The listing builds one solid part. Answer for the finished solid, in the listing's coordinates (mm). Coordinates: 2 decimals unless noted, no trailing zeros. Loops run counter-clockwise (first coordinate to the right, second up) from the corner with the lowest first, then second, coordinate; pieces in that order, holes last. Notation, with made-up numbers: (60, -32) - (97, -32) arc R7 ccw to (97, -28) - close; hole circle Ø10 at (82.5, -13). An arc over 180 degrees is marked (long way). Put each result on its own line as item: value.
```python
from build123d import *

# Parameters (mm, degrees)
SKETCH1_W           = 31.75
SKETCH1_H           = 38.1
BOSS_EXTRUDE1_DEPTH = 3.175
SKETCH2_R           = 2.15265
CUT_EXTRUDE1_DEPTH  = 42.760604941
SKETCH3_R           = 9.525
CUT_EXTRUDE2_DEPTH  = 42.760604941


with BuildPart() as part:
    # Sketch1 → Boss-Extrude1 (new, symmetric)
    with BuildSketch(Plane(origin=(0, 0, 0), x_dir=(0, 0, -1), z_dir=(1, 0, 0))):
        with Locations((0, 19.05)):
            Rectangle(SKETCH1_W, SKETCH1_H)
    extrude(amount=BOSS_EXTRUDE1_DEPTH, both=True)

    # Sketch2 → Cut-Extrude1 (cut, through all)
    with BuildSketch(Plane(origin=(3.175, 0, 0), x_dir=(0, 0, -1), z_dir=(1, 0, 0))):
        with Locations((-12.7, 3.175)):
            Circle(SKETCH2_R)
        with Locations((-12.7, 34.925)):
            Circle(SKETCH2_R)
        with Locations((12.7, 3.175)):
            Circle(SKETCH2_R)
        with Locations((12.7, 34.925)):
            Circle(SKETCH2_R)
    extrude(amount=-CUT_EXTRUDE1_DEPTH, mode=Mode.SUBTRACT)

    # Sketch3 → Cut-Extrude2 (cut, through all)
    with BuildSketch(Plane(origin=(3.175, 0, 0), x_dir=(0, 0, -1), z_dir=(1, 0, 0))):
        with Locations((0, 19.05)):
            Circle(SKETCH3_R)
    extrude(amount=-CUT_EXTRUDE2_DEPTH, mode=Mode.SUBTRACT)


solid = part.part
```
1) Straight lines are drawn through the part: L1, parallel to Y at x = -1.5, z = -12.7; L2, parallel to Z at x = -2, y = 36.5 (3 decimals); L3, parallel to Z at x = -1.25, y = 36 (3 decimals). For each, find the intervals that lie inside material, in ascending order. Write a range as [from, to].
Found:
L1: y = [0, 1.02], [5.33, 32.77], [37.08, 38.1]
L2: z = [-15.875, -14.167], [-11.233, 11.233], [14.167, 15.875]
L3: z = [-15.875, -14.565], [-10.835, 10.835], [14.565, 15.875]
2) For a pull along Y with two mould halves and no side action, classify faces 1 (the face through (0.04, 9.75, 2.06)), 2 (the face through (0, 38.1, 0)), 3 (the face through (0, 0, 0)), 4 (the face through (0, 19, -15.875)) as pulls with the +Y half, pulls with the -Y half, needs draft (parallel to the pull), parting line crosses it, or undercut.
Found:
face 1: undercut
face 2: pulls with the +Y half
face 3: pulls with the -Y half
face 4: needs draft
3) The part is cut by section B-B (y = 19.05). Give the vertices of the cut face in (x, z) (3 decimals), and give its area (3 significant figures).
Found:
outline: (-3.175, -15.875) - (3.175, -15.875) - (3.175, -9.525) - (-3.175, -9.525) - close; (-3.175, 9.525) - (3.175, 9.525) - (3.175, 15.875) - (-3.175, 15.875) - close
area: 80.6 mm^2
4) The part is cut by section D-D (x = 0.5). Give the vertices of the cut face in (y, z) (3 decimals), and give its area (3 significant figures).
Found:
outline: (0, -15.875) - (38.1, -15.875) - (38.1, 15.875) - (0, 15.875) - close; hole circle Ø4.305 at (3.175, -12.7); hole circle Ø4.305 at (3.175, 12.7); hole circle Ø19.05 at (19.05, 0); hole circle Ø4.305 at (34.925, -12.7); hole circle Ø4.305 at (34.925, 12.7)
area: 866 mm^2
5) The part is cut by section C-C (z = 0). Give the vertices of the cut face in (x, y) (3 decimals), and give its area (3 significant figures).
Found:
outline: (-3.175, 0) - (3.175, 0) - (3.175, 9.525) - (-3.175, 9.525) - close; (-3.175, 28.575) - (3.175, 28.575) - (3.175, 38.1) - (-3.175, 38.1) - close
area: 121 mm^2
6) The part is cut by section A-A (z = -12.7). Give the vertices of the cut face in (x, y) (3 decimals).
Found:
outline: (-3.175, 0) - (3.175, 0) - (3.175, 1.022) - (-3.175, 1.022) - close; (-3.175, 5.328) - (3.175, 5.328) - (3.175, 32.772) - (-3.175, 32.772) - close; (-3.175, 37.078) - (3.175, 37.078) - (3.175, 38.1) - (-3.175, 38.1) - close
